Input: part model. Units: mm. Frame: model coordinates. A direction names the side the tool comes from. Give positions to 0.01 mm unless a question says otherwise; leave off trailing zeros. Loops run counter-clockwise (first coordinate to the right, second up) from the corner with the lowest first, then second, coordinate; pieces in that order, holes last. Notation, with made-up numbers: M -20,-29.75 L 25,-29.75 A13 cw 25,-24.75 Z; hole C -15,22.5 d4. An arc over 180 degrees is marked long. Answer as a JSON object with one key per item and string values. Group by question number.
```python
from build123d import *

# Parameters (mm, degrees)
ESQUISSE1_R        = 1.75
BOSS_EXTRU_1_DEPTH = 2
BOSS_EXTRU_2_START = -0.25
ESQUISSE3_R        = 1.75
BOSS_EXTRU_2_DEPTH = 0.25
ESQUISSE2_R        = 1
BOSS_EXTRU_3_DEPTH = 8
CONG_1_R           = 0.1


with BuildPart() as part:
    # Esquisse1 → Boss.-Extru.1 (new body)
    with BuildSketch(Plane.XY):
        Circle(ESQUISSE1_R)
        Polygon((0.577350269, -1), (1.154700538, 0), (0.577350269, 1), (-0.577350269, 1), (-1.154700538, 0), (-0.577350269, -1), align=None, mode=Mode.SUBTRACT)
    extrude(amount=BOSS_EXTRU_1_DEPTH)

    # Esquisse3 → Boss.-Extru.2 (add)
    with BuildSketch(Plane.XY.offset(2).offset(BOSS_EXTRU_2_START)):
        Circle(ESQUISSE3_R)
    extrude(amount=BOSS_EXTRU_2_DEPTH)

    # Esquisse2 → Boss.-Extru.3 (add)
    with BuildSketch(Plane.XY.offset(2)):
        Circle(ESQUISSE2_R)
    extrude(amount=BOSS_EXTRU_3_DEPTH)

    # Congé1
    cong_1_edges = [part.edges().sort_by_distance(p)[0] for p in [
        (-1.75, 0, 0),
        (-1, 0, 2),
        (-1.75, 0, 2),
    ]]
    fillet(cong_1_edges, radius=CONG_1_R)


solid = part.part
```
1. Section C-C (z = 6.75). Output: boundary loops of the cut face in (x, y), then the cut area to 3 significant figures.
2. Reachability of faces 4 (the flat face through (-0.87, -0.49, 0.86)), 5 (the cylindrical face through (1.617, -0.67, 0.987)) from +Z, -Z, +X, -X, +Y, -Y: full face, straight path, thin tool, end or side. Return the list, or none.
3. First-contact query: P1, Ø1.5, axis at x = -0.5, z = 3.5, coming from the -Y side; P2, Ø1, axis at y = 0, z = 7.5, coming from the -X side. Flat tips, straight axial feed; report the tip coordinate or a pass-through.
4. Section A-A (z = 1.5). Output: boundary loops of the cut face in (x, y).
5. Mould query, pull axis Y, two halves, no side actions, for faces 1 (the flat face through (-0.86, 0.51, 0.86)), 2 (the flat face through (0, 0, 10)), 3 (the cylindrical face through (0, -1, 6)). Classes: pulls with the +Y half, pulls with the -Y half, needs draft (parallel to the pull), parting line crosses it, or undercut.
6. Material intervals for L1, parallel to Z at x = -1.45, y = 0.4; L2, parallel to Y at x = 1.1, z = 1.25; L3, parallel to Z at x = -0.2, y = -0.45, sorted ascending.
7. Section B-B (x = 0). Output: boundary loops of the cut face in (y, z), then the cut area to 3 significant figures.
Geometry results:
{
 "1": {"outline": "C 0,0 d2", "area": "3.14 mm2"},
 "2": {"face 4": "-Z", "face 5": "+Z, -Z"},
 "3": {"P1": "y = -1", "P2": "x = -1"},
 "4": {"outline": "C 0,0 d3.5; hole M -1.15,0 L -0.58,-1 L 0.58,-1 L 1.15,0 L 0.58,1 L -0.58,1 Z"},
 "5": {"face 1": "undercut", "face 2": "needs draft", "face 3": "parting line crosses it"},
 "6": {"L1": "0 to 2", "L2": "-1.36 to -0.09, 0.09 to 1.36", "L3": "1.75 to 10"},
 "7": {"outline": "M -1.75,0.1 A0.1 ccw -1.65,0 L -1,0 L -1,1.75 L 1,1.75 L 1,0 L 1.65,0 A0.1 ccw 1.75,0.1 L 1.75,1.9 A0.1 ccw 1.65,2 L 1.1,2 A0.1 cw 1,2.1 L 1,10 L -1,10 L -1,2.1 A0.1 cw -1.1,2 L -1.65,2 A0.1 ccw -1.75,1.9 Z", "area": "19.5 mm2"}
}
